```python
from build123d import *
from build123d.topology import SkipClean

# Parameters (mm, degrees)
SKETCH_1_R          = 7.5
SKETCH_1_R_2        = 4
EXTRUDE_1_DEPTH     = 2
FILLET_1_R          = 10
EXTRUDE_START       = 3
SKETCH_2_R          = 4
EXTRUDE_2_DEPTH     = 3
CUT_EXTRUDE_1_DEPTH = 52.537192438


with BuildPart() as part:
    # Эскиз1 → Бобышка-Вытянуть1 (new body)
    # profile 1 of 6: a face of its own
    with BuildSketch(Plane.XY):
        with Locations((-38.385066635, -15.426902632)):
            Circle(SKETCH_1_R)
        with Locations((-38.385066635, -15.426902632)):
            Circle(SKETCH_1_R_2, mode=Mode.SUBTRACT)
    # profile 2 of 6: a face of its own
    with BuildSketch(Plane.XY):
        with BuildLine():
            ThreePointArc((-20, -7.5), (-27.047694656, -2.565151075), (-24.820907073, 5.745333323))
            Line((-24.820907073, 5.745333323), (-43.205973708, -9.681569309))
            ThreePointArc((-43.205973708, -9.681569309), (-35.215429672, -8.62959423), (-30.885066635, -15.426902632))
            ThreePointArc((-30.885066635, -15.426902632), (-31.587758232, -18.596539596), (-33.564159562, -21.172235956))
            Line((-33.564159562, -21.172235956), (-17.270223243, -7.5))
            Line((-17.270223243, -7.5), (-20, -7.5))
        make_face()
    # profile 3 of 6: a face of its own
    with BuildSketch(Plane.XY):
        with Locations((-20, 0)):
            Circle(SKETCH_1_R)
        with Locations((-20, 0)):
            Circle(SKETCH_1_R_2, mode=Mode.SUBTRACT)
    # profile 4 of 6: a face of its own
    with BuildSketch(Plane.XY):
        with BuildLine():
            Line((-20, -7.5), (-17.270223243, -7.5))
            Line((-17.270223243, -7.5), (-15.179092927, -5.745333323))
            ThreePointArc((-15.179092927, -5.745333323), (-17.434848925, -7.047694656), (-20, -7.5))
        make_face()
    # profile 5 of 6: a face of its own
    with BuildSketch(Plane.XY):
        with BuildLine():
            ThreePointArc((0, -7.5), (-7.5, 0), (0, 7.5))
            Line((0, 7.5), (-20, 7.5))
            ThreePointArc((-20, 7.5), (-14.696699141, 5.303300859), (-12.5, 0))
            ThreePointArc((-12.5, 0), (-13.202691597, -3.169636963), (-15.179092927, -5.745333323))
            Line((-15.179092927, -5.745333323), (-17.270223243, -7.5))
            Line((-17.270223243, -7.5), (0, -7.5))
        make_face()
    # profile 6 of 6: a face of its own
    with BuildSketch(Plane.XY):
        Circle(SKETCH_1_R)
        Circle(SKETCH_1_R_2, mode=Mode.SUBTRACT)
    extrude(amount=EXTRUDE_1_DEPTH)

    # Скругление1
    fillet_1_edges = [part.edges().sort_by_distance(p)[0] for p in [
        (-17.270223243, -7.5, 1),
    ]]
    fillet(fillet_1_edges, radius=FILLET_1_R)

    # Эскиз2 → Бобышка-Вытянуть2 (add)
    with SkipClean():  # the faces are left unmerged after this step: merging them gives an invalid solid
        with BuildSketch(Plane(origin=(0, 0, 0), x_dir=(-1, 0, 0), z_dir=(0, 0, -1)).offset(EXTRUDE_START)):
            with BuildLine():
                Line((0, -7.5), (15, -7.5))
                Line((15, -7.5), (15, 7.5))
                Line((15, 7.5), (0, 7.5))
                ThreePointArc((0, 7.5), (-7.5, 0), (0, -7.5))
            make_face()
            Circle(SKETCH_2_R, mode=Mode.SUBTRACT)
        extrude(amount=-EXTRUDE_2_DEPTH)

    # Эскиз4 → Вырез-Вытянуть1 (cut, through all)
    with BuildSketch(Plane.XY.offset(2)):
        with BuildLine():
            Line((-23.955125919, 0.597477168), (-38.286666374, -11.428113142))
            ThreePointArc((-38.286666374, -11.428113142), (-35.52206113, -12.633481884), (-34.385066635, -15.426902632))
            ThreePointArc((-34.385066635, -15.426902632), (-34.396300931, -15.726482609), (-34.429940716, -16.024379801))
            Line((-34.429940716, -16.024379801), (-20.098400261, -3.99878949))
            ThreePointArc((-20.098400261, -3.99878949), (-23.064177772, -2.571150439), (-23.955125919, 0.597477168))
        make_face()
        with BuildLine():
            Line((-2.645751311, 3), (-17.354248689, 3))
            ThreePointArc((-17.354248689, 3), (-16.354248689, 1.645751311), (-16, 0))
            ThreePointArc((-16, 0), (-16.354248689, -1.645751311), (-17.354248689, -3))
            Line((-17.354248689, -3), (-2.645751311, -3))
            ThreePointArc((-2.645751311, -3), (-4, 0), (-2.645751311, 3))
        make_face()
    extrude(amount=-CUT_EXTRUDE_1_DEPTH, mode=Mode.SUBTRACT)


solid = part.part
```
Geometry: final body of the model. Coordinates: model frame, mm. A direction names the side the tool comes from. Coordinates: 2 decimals unless noted, no trailing zeros. Order: outer loops, then holes, each group sorted by start corner. A loop starts at its lowest first (then second) coordinate and runs counter-clockwise, first axis right, second up. Notation, with made-up numbers: (57.25, 28.5) -> (102.25, 28.5) arc R23 cw to (102.25, 52.5) -> close; hole circle Ø6 at (71, 29). An arc over 180 degrees is marked (long way). Write each question's results on one line, items separated by ' | '. Start each with the question number.
1) First-contact query: pin 1 (3 mm diameter, centred on x = 0.5, z = -1, fed in from -Y); pin 2 (1 mm diameter, centred on x = -16, y = 1, fed in from -Z); pin 3 (6 mm diameter, centred on x = -19, y = -11, fed in from +Z); pin 4 (2 mm diameter, centred on x = -27, y = 1.5, fed in from -Z). Flat tips, straight axial feed; report the tip coordinate or a pass-through.
2) Cut plane C-C, the plane y = 2. Output: boundary loops of the cut face in (x, z), and give its area (3 significant figures).
3) Cut plane A-A, the plane x = -10. Output: boundary loops of the cut face in (y, z).
4) Mould query, pull axis X, two halves, no side actions, for faces 3 (the flat face through (-15, 5, -2)), 4 (the flat face through (-10, -3, 0)), 5 (the cylindrical face through (-44.235, -20.12, 0.986)). Classes: released by +X, released by -X, zero draft, split by the parting line, or undercut.
5) Cut plane D-D, the plane z = -2.4. Output: boundary loops of the cut face in (x, y).
6) Cut plane B-B, the plane z = 0.85. Output: boundary loops of the cut face in (x, y), and give its area (3 significant figures).
7) Material intervals for line 1 along Y through (x, z) = (0, -1.9); line 2 along Y through (x, z) = (-7.5, 0.1); line 3 along Z through (x, y) = (-22, 5), sorted ascending.
8) Set-up query: faces 1 (the flat face through (-19, -5, 2)), 2 (the cylindrical face through (-18.652, -3.766, 0.986)). Return all of +Z, -Z, +X, -X, +Y, -Y with unobstructed straight access to the full face (end or side cutting, diameter ignored); none if empty.
Checks:
1) pin 1: y = -7.5 | pin 2: through | pin 3: z = 2 | pin 4: z = 0
2) outline: (-29.28, 0) -> (-23.46, 0) -> (-23.46, 2) -> (-29.28, 2) -> close; (3.46, -3) -> (7.23, -3) -> (7.23, 2) -> (3.46, 2) -> close | area: 30.5 mm^2
3) outline: (-7.5, -3) -> (-3, -3) -> (-3, 2) -> (-7.5, 2) -> close; (3, -3) -> (7.5, -3) -> (7.5, 2) -> (3, 2) -> close
4) face 3: released by -X | face 4: undercut | face 5: split by the parting line
5) outline: (-15, -7.5) -> (0, -7.5) arc R7.5 ccw to (0, 7.5) -> (-15, 7.5) -> (-15, 3) -> (-2.65, 3) arc R4 cw (long way) to (-2.65, -3) -> (-15, -3) -> close
6) outline: (-43.21, -9.68) arc R7.5 ccw to (-33.56, -21.17) -> (-20.06, -9.84) arc R10 cw to (-13.63, -7.5) -> (0, -7.5) arc R7.5 ccw to (0, 7.5) -> (-20, 7.5) arc R7.5 ccw to (-24.82, 5.75) -> close; hole (-38.29, -11.43) arc R4 ccw (long way) to (-34.43, -16.02) -> (-20.1, -4) arc R4 ccw to (-17.35, -3) -> (-2.65, -3) arc R4 ccw (long way) to (-2.65, 3) -> (-17.35, 3) arc R4 ccw to (-23.96, 0.6) -> close | area: 509 mm^2
7) line 1: -7.5 to -4, 4 to 7.5 | line 2: -7.5 to -3, 3 to 7.5 | line 3: 0 to 2
8) face 1: +Z, +X, -X, +Y, -Y | face 2: +Z, -Z
